```python
from build123d import *

# Parameters (mm, degrees)
SKETCH_2_W          = 1.7
SKETCH_2_H          = 0.6
SKETCH_2_W_2        = 0.6
SKETCH_2_H_2        = 1.7
CUT_EXTRUDE_1_DEPTH = 0.5
FILLET_1_R          = 0.8


with BuildPart() as part:
    # 草图1 → 旋转1 (revolve)
    with BuildSketch(Plane.XY):
        Polygon((0, 0), (0, 2.95), (2.7, 2.95), (2.7, 1.75), (6.7, 1.75), (6.7, 0), align=None)
    revolve(axis=Axis((6.7, 0, 0), (-1, 0, 0)))

    # 草图2 → 切除-拉伸1 (cut)
    with BuildSketch(Plane.ZY):
        with Locations((1.15, 0)):
            Rectangle(SKETCH_2_W, SKETCH_2_H)
        with Locations((0, -1.15)):
            Rectangle(SKETCH_2_W_2, SKETCH_2_H_2)
        Rectangle(SKETCH_2_W_2, SKETCH_2_H)
        with Locations((0, 1.15)):
            Rectangle(SKETCH_2_W_2, SKETCH_2_H_2)
        with Locations((-1.15, 0)):
            Rectangle(SKETCH_2_W, SKETCH_2_H)
    extrude(amount=-CUT_EXTRUDE_1_DEPTH, mode=Mode.SUBTRACT)

    # 圆角1
    fillet_1_edges = [part.edges().sort_by_distance(p)[0] for p in [
        (2.7, -2.95, 0),
        (0, -2.95, 0),
    ]]
    fillet(fillet_1_edges, radius=FILLET_1_R)


solid = part.part
```
Model file for the job. Use its own axes, mm. A direction names the side the tool comes from. Coordinates: 2 decimals unless noted, no trailing zeros. Loops run counter-clockwise (first coordinate to the right, second up) from the corner with the lowest first, then second, coordinate; pieces in that order, holes last. Notation, with made-up numbers: (42, -38) -> (50, -38) arc R28 ccw to (50, -20) -> close; hole circle Ø1 at (-20, 66.5). An arc over 180 degrees is marked (long way). Answer as a JSON object with one key per item and string values.
Q1. Flat gauge pins, fed straight in: P1, Ø2, axis at x = 3.5, y = 1, coming from the +Z side; P2, Ø1, axis at x = 3.5, z = 1, coming from the -Y side; P3, Ø0.6, axis at x = 0, z = 1, coming from the +Y side; P4, Ø3, axis at y = -0.5, z = 1, coming from the -X side. Where does each tip first touch, or does it go through?
Report:
{"P1": "stops at z = 2.53", "P2": "stops at y = -1.68", "P3": "stops at y = 2.61", "P4": "stops at x = 0"}
Q2. Cut at C-C (x = 4.5). List the corners of the cut face in (y, z).
Report:
{"outline": "circle Ø3.5 at (0, 0)"}
Q3. Probe probe 1 along X at (y, z) = (-1.2, 1.45); probe 2 along Y at (x, z) = (1, -0.25); probe 3 along Z at (x, y) = (2, -2.35). List the from-to ranges inside material, lowest first.
Report:
{"probe 1": "x = 0 to 2.7", "probe 2": "y = -2.94 to 2.94", "probe 3": "z = -1.77 to 1.77"}
Q4. Pull direction Y, two halves, no side cores. Call faces 3 (the flat face through (0.5, 0, 0)), 4 (the flat face through (6.7, 0, 0)), 5 (the cylindrical face through (1.358, -2.947, -0.13)): released by +Y, released by -Y, zero draft, split by the parting line, or undercut.
Report:
{"face 3": "undercut", "face 4": "zero draft", "face 5": "split by the parting line"}
Q5. Cut at A-A (z = 0). List the corners of the cut face in (x, y), and give its area (3 significant figures).
Report:
{"outline": "(0, -2.15) arc R0.8 ccw to (0.8, -2.95) -> (1.9, -2.95) arc R0.8 ccw to (2.7, -2.15) -> (2.7, -1.75) -> (6.7, -1.75) -> (6.7, 1.75) -> (2.7, 1.75) -> (2.7, 2.15) arc R0.8 ccw to (1.9, 2.95) -> (0.8, 2.95) arc R0.8 ccw to (0, 2.15) -> (0, 2) -> (0.5, 2) -> (0.5, -2) -> (0, -2) -> close", "area": "27.4 mm2"}
Q6. 3-axis set-ups, long thin cutter, end or side, ignore diameter. For faces 1 (the cylindrical face through (4.728, 1.617, 0.67)), 2 (the flat face through (0, -0.45, 0.45)): which of +Z, -Z, +X, -X, +Y, -Y reach the whole face in a straight line?
Report:
{"face 1": "+X", "face 2": "+Z, -Z, -X, +Y, -Y"}
